Autodesk Inventor part; units mm, degrees
ref_plane "YZ Plane" through (0, 0, 0) normal (1, 0, 0) x (0, 1, 0)
ref_plane "XZ Plane" through (0, 0, 0) normal (0, 1, 0) x (-1, 0, 0)
ref_plane "XY Plane" through (0, 0, 0) normal (0, 0, 1) x (1, 0, 0)
sketch "Sketch1" plane through (0, 0, 0) normal (1, 0, 0) x (0, 1, 0)
  line L0 (0, 0) -> (0, -1.725)
  line L1 (0, -1.725) -> (0.86, -1.725)
  line L2 (0.86, -1.725) -> (0.86, -3.005)
  line L3 (0.86, -3.005) -> (6.36, -3.005)
  line L4 (6.36, -3.005) -> (6.36, -3.505)
  line L5 (6.36, -3.505) -> (16.28, -3.505)
  line L6 (16.28, -3.505) -> (18.6408, -4.815)
  line L7 (18.6408, -4.815) -> (34.9681, -4.815)
  line L8 (34.9681, -4.815) -> (35.9725, -3.005)
  line L9 (35.9725, -3.005) -> (37.64, -3.005)
  line L10 (37.64, -3.005) -> (37.64, 0)
  line L11 (37.64, 0) -> (0, 0)
  dimension "d0" = 1.725
  dimension "d1" = 0.86
  dimension "d2" = 1.28
  dimension "d3" = 90
  dimension "d4" = 5.5
  dimension "d5" = 0.5
  dimension "d6" = 9.92
  dimension "d7" = 4.815
  dimension "d8" = 37.64
revolve "Revolution1" add sketch "Sketch1" angle 360 about axis through (0, 37.64, 0) along (0, -1, 0)
properties part number "00_RS_Pro_Micrometer_small"
Design review of the part built by this model. Coordinates are the model's own, in mm. A direction names the side the tool comes from. Give positions to 0.01 mm unless a question says otherwise; leave off trailing zeros. Write each loop counter-clockwise with the first axis right and the second up, starting at its lowest first coordinate (ties: lowest second). Pieces come first, ordered by that corner, then holes.
(1) Add section C-C (y = 12.5). Give the boundary of the cut face in (x, z) (3 decimals), and give its area (3 significant figures).
Checked values:
outline: circle Ø7.01 at (0, 0)
area: 38.6 mm2
(2) Add section B-B (x = 0). Give the boundary of the cut face in (y, z) (1 decimal).
Checked values:
outline: (0, -1.7) - (0.9, -1.7) - (0.9, -3) - (6.4, -3) - (6.4, -3.5) - (16.3, -3.5) - (18.6, -4.8) - (35, -4.8) - (36, -3) - (37.6, -3) - (37.6, 3) - (36, 3) - (35, 4.8) - (18.6, 4.8) - (16.3, 3.5) - (6.4, 3.5) - (6.4, 3) - (0.9, 3) - (0.9, 1.7) - (0, 1.7) - close
(3) Add section A-A (z = 0). Give the boundary of the cut face in (x, y) (1 decimal).
Checked values:
outline: (-4.8, 18.6) - (-3.5, 16.3) - (-3.5, 6.4) - (-3, 6.4) - (-3, 0.9) - (-1.7, 0.9) - (-1.7, 0) - (1.7, 0) - (1.7, 0.9) - (3, 0.9) - (3, 6.4) - (3.5, 6.4) - (3.5, 16.3) - (4.8, 18.6) - (4.8, 35) - (3, 36) - (3, 37.6) - (-3, 37.6) - (-3, 36) - (-4.8, 35) - close
(4) Wall thickness on line 1 along Z through (x, y) = (-0.25, 34.5); line 2 along Z through (x, y) = (1.75, 18); line 3 along X through (y, z) = (30, 4.25): over which ranges is each line inside the solid? List them lowest first.
Checked values:
line 1: z = -4.81 to 4.81
line 2: z = -4.1 to 4.1
line 3: x = -2.26 to 2.26
(5) Tool access review of faces 1 (the face through (-0.903, 36.818, -2.866)), 2 (the face through (4.7, 26.92, 1.04)), 3 (the face through (-1.71, 0.44, 0.22)): name each direction out of +Z, -Z, +X, -X, +Y, -Y from which nothing blocks a thin tool from reaching the whole face with its end or side.
Checked values:
face 1: +Y
face 2: +Y, -Y
face 3: -Y
(6) Clearance check with flat-ended pins moving along their axes: pin 1 Ø2 at (x, y) = (-3.5, 7.5) entering from -Z; pin 2 Ø1 at (x, y) = (-2, 17) entering from +Z; pin 3 Ø2 at (x, y) = (2, 9) entering from +Z. State where each tip first meets the part, or that it passes through.
Checked values:
pin 1: stops at z = -2.46
pin 2: stops at z = 3.76
pin 3: stops at z = 3.36
